Model file for the job. Use its own axes, mm. Coordinates: 2 decimals unless noted, no trailing zeros. Order: outer loops, then holes, each group sorted by start corner. A loop starts at its lowest first (then second) coordinate and runs counter-clockwise, first axis right, second up.
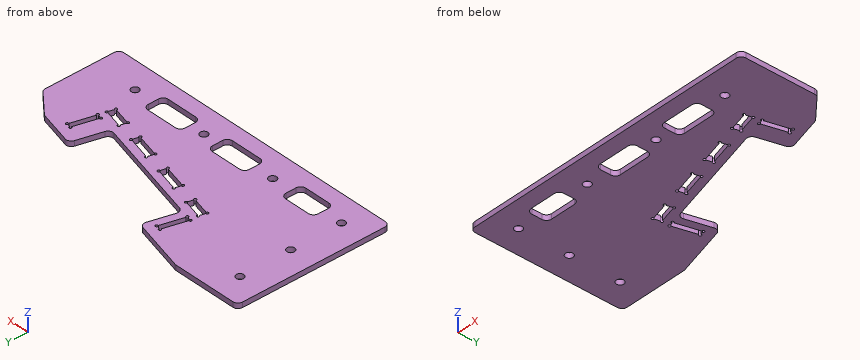
from build123d import *

# Parameters (mm, degrees)
SKETCH_1_W           = 130
SKETCH_1_H           = 60
SKETCH_1_R           = 1.5
EXTRUDE_1_DEPTH      = 2
CUT_EXTRUDE_1_DEPTH  = 3
CUT_EXTRUDE_2_DEPTH  = 3
CUT_EXTRUDE_5_DEPTH  = 10
CUT_EXTRUDE_6_DEPTH  = 3
FILLET_1_R           = 2
CUT_EXTRUDE_7_DEPTH  = 3
CUT_EXTRUDE_8_DEPTH  = 10
CUT_EXTRUDE_9_DEPTH  = 10
EXTRUDE_2_DEPTH      = 2
SKETCH_9_R           = 0.5
CUT_EXTRUDE_10_DEPTH = 10


with BuildPart() as part:
    # 草图1 → 凸台-拉伸1 (new body)
    with BuildSketch(Plane.XY):
        with Locations((65, 30)):
            Rectangle(SKETCH_1_W, SKETCH_1_H)
        with Locations((10, 10)):
            Circle(SKETCH_1_R, mode=Mode.SUBTRACT)
        with Locations((10, 30)):
            Circle(SKETCH_1_R, mode=Mode.SUBTRACT)
        with Locations((10, 50)):
            Circle(SKETCH_1_R, mode=Mode.SUBTRACT)
        with Locations((40, 10)):
            Circle(SKETCH_1_R, mode=Mode.SUBTRACT)
        with Locations((70, 10)):
            Circle(SKETCH_1_R, mode=Mode.SUBTRACT)
        with Locations((100, 10)):
            Circle(SKETCH_1_R, mode=Mode.SUBTRACT)
    extrude(amount=EXTRUDE_1_DEPTH)

    # 草图2 → 切除-拉伸1 (cut, through all)
    with BuildSketch(Plane.XY.offset(2)):
        Polygon((27, 60), (130, 32.40123318), (130, 60), align=None)
    extrude(amount=-CUT_EXTRUDE_1_DEPTH, mode=Mode.SUBTRACT)

    # 草图3 → 切除-拉伸2 (cut, through all)
    with BuildSketch(Plane.XY.offset(2)):
        Polygon((49.071405131, 54.085984819), (93.50399314, 42.180308745), (89.880526509, 28.657347177), (45.447938499, 40.563023251), align=None)
    extrude(amount=-CUT_EXTRUDE_2_DEPTH, mode=Mode.SUBTRACT)

    # 草图4 → 切除-拉伸5 (cut)
    with BuildSketch(Plane.XY.offset(2)):
        Polygon((98.74723483, 36.634281646), (96.159044379, 26.975023383), (98.090896032, 26.457385293), (100.679086483, 36.116643556), align=None)
        Polygon((45.138351471, 50.99873865), (42.55016102, 41.339480387), (40.618309368, 41.857118477), (43.206499819, 51.51637674), align=None)
    extrude(amount=-CUT_EXTRUDE_5_DEPTH, mode=Mode.SUBTRACT)

    # 草图5 → 切除-拉伸6 (cut, through all)
    with BuildSketch(Plane.XY.offset(2)):
        Polygon((130, 20), (130, 32.40123318), (108.287273653, 38.21914067), (118, 30.069195574), (118, 0), (130, 0), align=None)
    extrude(amount=-CUT_EXTRUDE_6_DEPTH, mode=Mode.SUBTRACT)

    # 圆角1
    fillet_1_edges = [part.edges().sort_by_distance(p)[0] for p in [
        (118, 30.069195574, 1),
        (108.287273653, 38.21914067, 1),
        (118, 0, 1),
        (27, 60, 1),
        (45.447938499, 40.563023251, 1),
        (49.071405131, 54.085984819, 1),
        (93.50399314, 42.180308745, 1),
        (89.880526509, 28.657347177, 1),
        (0, 60, 1),
        (0, 0, 1),
    ]]
    fillet(fillet_1_edges, radius=FILLET_1_R)

    # 草图6 → 切除-拉伸7 (cut)
    with BuildSketch(Plane(origin=(0, 0, 0), x_dir=(-1, 0, 0), z_dir=(0, 0, -1))):
        with BuildLine():
            Line((-78, 14), (-90, 14))
            ThreePointArc((-90, 14), (-91.414213562, 13.414213562), (-92, 12))
            Line((-92, 12), (-92, 8))
            ThreePointArc((-92, 8), (-91.414213562, 6.585786438), (-90, 6))
            Line((-90, 6), (-78, 6))
            ThreePointArc((-78, 6), (-76.585786438, 6.585786438), (-76, 8))
            Line((-76, 8), (-76, 12))
            ThreePointArc((-76, 12), (-76.585786438, 13.414213562), (-78, 14))
        make_face()
        with BuildLine():
            Line((-50, 14), (-62, 14))
            ThreePointArc((-62, 14), (-63.414213562, 13.414213562), (-64, 12))
            Line((-64, 12), (-64, 8))
            ThreePointArc((-64, 8), (-63.414213562, 6.585786438), (-62, 6))
            Line((-62, 6), (-50, 6))
            ThreePointArc((-50, 6), (-48.585786438, 6.585786438), (-48, 8))
            Line((-48, 8), (-48, 12))
            ThreePointArc((-48, 12), (-48.585786438, 13.414213562), (-50, 14))
        make_face()
        with BuildLine():
            Line((-20, 14), (-30, 14))
            ThreePointArc((-30, 14), (-31.414213562, 13.414213562), (-32, 12))
            Line((-32, 12), (-32, 8))
            ThreePointArc((-32, 8), (-31.414213562, 6.585786438), (-30, 6))
            Line((-30, 6), (-20, 6))
            ThreePointArc((-20, 6), (-18.585786438, 6.585786438), (-18, 8))
            Line((-18, 8), (-18, 12))
            ThreePointArc((-18, 12), (-18.585786438, 13.414213562), (-20, 14))
        make_face()
    extrude(amount=-CUT_EXTRUDE_7_DEPTH, mode=Mode.SUBTRACT)

    # 草图7 → 切除-拉伸8 (cut)
    with BuildSketch(Plane.XY.offset(2)):
        Polygon((97.314438897, 23.559607814), (89.944424842, 25.534397129), (89.167967707, 22.63661965), (96.537981761, 20.661830336), align=None)
        Polygon((81.440561097, 24.70717201), (82.217018232, 27.604949489), (72.915152525, 30.097376894), (72.138695389, 27.199599415), align=None)
        Polygon((64.411288779, 29.270151776), (65.187745914, 32.167929255), (55.885880207, 34.660356659), (55.109423072, 31.76257918), align=None)
        Polygon((47.382016462, 33.833131541), (48.158473597, 36.73090902), (40.788459542, 38.705698334), (40.012002407, 35.807920855), align=None)
    extrude(amount=-CUT_EXTRUDE_8_DEPTH, mode=Mode.SUBTRACT)

    # 草图8 → 切除-拉伸9 (cut)
    with BuildSketch(Plane.XY.offset(2)):
        Polygon((98.726021627, 36.671023993), (96.122302033, 26.95381018), (98.112109235, 26.420642947), (100.715828829, 36.13785676), align=None)
        Polygon((97.351181243, 23.580821018), (89.923211639, 25.571139475), (89.131225361, 22.615406446), (96.559194965, 20.625087989), align=None)
        Polygon((81.4617743, 24.670429664), (82.253760578, 27.626162693), (72.893939321, 30.13411924), (72.101953043, 27.178386211), align=None)
        Polygon((64.432501982, 29.23340943), (65.22448826, 32.189142458), (55.864667004, 34.697099005), (55.072680726, 31.741365977), align=None)
        Polygon((47.403229665, 33.796389195), (48.195215943, 36.752122223), (40.767246339, 38.74244068), (39.975260061, 35.786707652), align=None)
        Polygon((43.185286615, 51.553119086), (40.581567022, 41.835905273), (42.571374224, 41.302738041), (45.175093818, 51.019951853), align=None)
    extrude(amount=-CUT_EXTRUDE_9_DEPTH, mode=Mode.SUBTRACT)

    # 草图10 → 凸台-拉伸2 (add)
    with BuildSketch(Plane.XY.offset(2)):
        Polygon((40.767246339, 38.74244068), (48.195215943, 36.752122223), (48.169334038, 36.65552964), (40.741364434, 38.645848097), align=None)
        Polygon((39.975260061, 35.786707652), (47.403229665, 33.796389195), (47.42911157, 33.892981777), (40.001141965, 35.883300234), align=None)
        Polygon((55.864667004, 34.697099005), (55.838785099, 34.600506422), (65.196979694, 32.092985738), (65.222861598, 32.189578321), align=None)
        Polygon((64.432501982, 29.23340943), (55.072680726, 31.741365977), (55.09856263, 31.837958559), (64.458383887, 29.330002012), align=None)
        Polygon((72.893939321, 30.13411924), (82.253760578, 27.626162693), (82.227878673, 27.52957011), (72.868057417, 30.037526657), align=None)
        Polygon((81.4617743, 24.670429664), (72.101953043, 27.178386211), (72.127834948, 27.274978794), (81.487656204, 24.767022247), align=None)
        Polygon((89.923211639, 25.571139475), (97.351181243, 23.580821018), (97.325299338, 23.484228435), (89.897329734, 25.474546892), align=None)
        Polygon((96.559194965, 20.625087989), (89.131225361, 22.615406446), (89.157107265, 22.711999029), (96.585076869, 20.721680572), align=None)
        Polygon((98.726021627, 36.671023993), (96.122302033, 26.95381018), (96.218894616, 26.927928276), (98.82261421, 36.645142088), align=None)
        Polygon((100.715828829, 36.13785676), (98.112109235, 26.420642947), (98.015516653, 26.446524852), (100.619236247, 36.163738664), align=None)
        Polygon((43.185286615, 51.553119086), (40.581567022, 41.835905273), (40.658841088, 41.81519975), (43.262560682, 51.532413562), align=None)
        Polygon((45.175093818, 51.019951853), (42.571374224, 41.302738041), (42.494100158, 41.323443564), (45.097819751, 51.040657377), align=None)
    extrude(amount=-EXTRUDE_2_DEPTH)

    # 草图9 → 切除-拉伸10 (cut)
    with BuildSketch(Plane.XY.offset(2)):
        with Locations((43.185286615, 51.553119086)):
            Circle(SKETCH_9_R)
        with Locations((45.175093818, 51.019951853)):
            Circle(SKETCH_9_R)
        with Locations((40.581567022, 41.835905273)):
            Circle(SKETCH_9_R)
        with Locations((42.571374224, 41.302738041)):
            Circle(SKETCH_9_R)
        with Locations((40.767246339, 38.74244068)):
            Circle(SKETCH_9_R)
        with Locations((48.195215943, 36.752122223)):
            Circle(SKETCH_9_R)
        with Locations((39.975260061, 35.786707652)):
            Circle(SKETCH_9_R)
        with Locations((47.403229665, 33.796389195)):
            Circle(SKETCH_9_R)
        with Locations((55.864667004, 34.697099005)):
            Circle(SKETCH_9_R)
        with Locations((55.072680726, 31.741365977)):
            Circle(SKETCH_9_R)
        with Locations((65.22448826, 32.189142458)):
            Circle(SKETCH_9_R)
        with Locations((64.432501982, 29.23340943)):
            Circle(SKETCH_9_R)
        with Locations((72.101953043, 27.178386211)):
            Circle(SKETCH_9_R)
        with Locations((72.893939321, 30.13411924)):
            Circle(SKETCH_9_R)
        with Locations((82.253760578, 27.626162693)):
            Circle(SKETCH_9_R)
        with Locations((81.4617743, 24.670429664)):
            Circle(SKETCH_9_R)
        with Locations((89.131225361, 22.615406446)):
            Circle(SKETCH_9_R)
        with Locations((89.923211639, 25.571139475)):
            Circle(SKETCH_9_R)
        with Locations((97.351181243, 23.580821018)):
            Circle(SKETCH_9_R)
        with Locations((96.559194965, 20.625087989)):
            Circle(SKETCH_9_R)
        with Locations((96.122302033, 26.95381018)):
            Circle(SKETCH_9_R)
        with Locations((98.112109235, 26.420642947)):
            Circle(SKETCH_9_R)
        with Locations((98.726021627, 36.671023993)):
            Circle(SKETCH_9_R)
        with Locations((100.715828829, 36.13785676)):
            Circle(SKETCH_9_R)
    extrude(amount=-CUT_EXTRUDE_10_DEPTH, mode=Mode.SUBTRACT)


solid = part.part
Q1. Cut at A-A, the plane y = 10. Count the separate pieces of the cut face and the enclosed holes in it, plus the area to 3 significant figures.
Established:
separate pieces: 8
enclosed holes: 0
area: 120 mm2
Q2. Probe line 1 (Y direction, x = 53, z = 1.2); line 2 (Y direction, x = 22.5, z = 0.7); line 3 (Y direction, x = 9, z = 1.9). List the from-to ranges inside material, lowest first.
Established:
line 1: y = 0 to 6, 14 to 38.54
line 2: y = 0 to 6, 14 to 60
line 3: y = 0 to 8.88, 11.12 to 28.88, 31.12 to 48.88, 51.12 to 60
Q3. Cut at B-B, the plane x = 70. List the corners of the cut face in (y, z).
Established:
outline: (0, 0) - (8.5, 0) - (8.5, 2) - (0, 2) - close; (11.5, 0) - (33.98, 0) - (33.98, 2) - (11.5, 2) - close
Q4. Drop flat-ended pins along their axis: P1, Ø1.8, axis at x = 10, y = 10, coming from the -Z side; P2, Ø4, axis at x = 10, y = 50, coming from the -Z side. Give the stop position or say it passes through.
Established:
P1: passes through
P2: stops at z = 0
